from build123d import *

# Parameters (mm, degrees)
SCHIZZO1_R                   = 225
ESTRUSIONE_ESTRUSIONE1_DEPTH = 18
TAGLIO_ESTRUSIONE3_DEPTH     = 56
TAGLIO_ESTRUSIONE4_DEPTH     = 110


with BuildPart() as part:
    # Schizzo1 → Estrusione-Estrusione1 (new body)
    with BuildSketch(Plane.XY):
        Circle(SCHIZZO1_R)
    extrude(amount=ESTRUSIONE_ESTRUSIONE1_DEPTH)

    # Schizzo1<7> → Taglio-Estrusione3 (cut)
    with BuildSketch(Plane.XY):
        with BuildLine():
            Line((-11.65, 168.428927822), (-6.35, 168.428927822))
            ThreePointArc((-6.35, 168.428927822), (-3.175, 171.603927822), (0, 168.428927822))
            Line((0, 168.428927822), (0, 157.428927822))
            Line((0, 157.428927822), (11, 157.428927822))
            ThreePointArc((11, 157.428927822), (14.175, 154.253927822), (11, 151.078927822))
            Line((11, 151.078927822), (11, 145.778927822))
            ThreePointArc((11, 145.778927822), (14.175, 142.603927822), (11, 139.428927822))
            Line((11, 139.428927822), (0, 139.428927822))
            Line((0, 139.428927822), (0, 128.428927822))
            ThreePointArc((0, 128.428927822), (-3.175, 125.253927822), (-6.35, 128.428927822))
            Line((-6.35, 128.428927822), (-11.65, 128.428927822))
            ThreePointArc((-11.65, 128.428927822), (-14.825, 125.253927822), (-18, 128.428927822))
            Line((-18, 128.428927822), (-18, 139.428927822))
            Line((-18, 139.428927822), (-29, 139.428927822))
            ThreePointArc((-29, 139.428927822), (-32.175, 142.603927822), (-29, 145.778927822))
            Line((-29, 145.778927822), (-29, 151.078927822))
            ThreePointArc((-29, 151.078927822), (-32.175, 154.253927822), (-29, 157.428927822))
            Line((-29, 157.428927822), (-18, 157.428927822))
            Line((-18, 157.428927822), (-18, 168.428927822))
            ThreePointArc((-18, 168.428927822), (-14.825, 171.603927822), (-11.65, 168.428927822))
        make_face()
    extrude(amount=TAGLIO_ESTRUSIONE3_DEPTH, mode=Mode.SUBTRACT)

    # Schizzo1<8> → Taglio-Estrusione4 (cut)
    with BuildSketch(Plane.XY):
        with BuildLine():
            Line((-70.097292154, -124.331072178), (-64.797292154, -124.331072178))
            ThreePointArc((-64.797292154, -124.331072178), (-61.622292154, -121.156072178), (-58.447292154, -124.331072178))
            Line((-58.447292154, -124.331072178), (-58.447292154, -142.331072178))
            ThreePointArc((-58.447292154, -142.331072178), (-61.622292154, -145.506072178), (-64.797292154, -142.331072178))
            Line((-64.797292154, -142.331072178), (-70.097292154, -142.331072178))
            ThreePointArc((-70.097292154, -142.331072178), (-73.272292154, -145.506072178), (-76.447292154, -142.331072178))
            Line((-76.447292154, -142.331072178), (-76.447292154, -124.331072178))
            ThreePointArc((-76.447292154, -124.331072178), (-73.272292154, -121.156072178), (-70.097292154, -124.331072178))
        make_face()
    extrude(amount=TAGLIO_ESTRUSIONE4_DEPTH, mode=Mode.SUBTRACT)


solid = part.part
Here's how the part is built. I have some questions about the finished solid (model axes, mm). A direction names the side the tool comes from. Round coordinates to 2 decimals unless told otherwise and drop trailing zeros. Write each loop counter-clockwise with the first axis right and the second up, starting at its lowest first coordinate (ties: lowest second). Pieces come first, ordered by that corner, then holes.
1. Suppose I cut it at A-A (z = 8.5). State how many separate pieces and enclosed holes the cut face has, and give its area (3 significant figures).
2. Will these pins go through, and if not, where does the flat tip stop? pin 1 Ø5.5 at (y, z) = (132.5, 12) entering from -X; pin 2 Ø6 at (x, z) = (-106.5, 7.5) entering from -Y; pin 3 Ø5.5 at (y, z) = (-129.5, 6.5) entering from -X.
3. I need wall thicknesses on L1, parallel to Y at x = -30.5, z = 11.25; L2, parallel to X at y = 6.5, z = 1.25; L3, parallel to X at y = -126, z = 9. Which ranges of each line are inside material? Lowest first, please.
4. For faces 1 (the flat face through (-3, 3, 18)), 2 (the flat face through (-23, 139.429, 9)), which set-ups out of +Z, -Z, +X, -X, +Y, -Y let a thin tool reach every point of the face, with its end or its side?
5. Suppose I cut it at B-B (y = 85). List the corners of the cut face in (x, z) for me.
6. If we mould it in two halves opening along X, with no side actions, what happens to faces 3 (the cylindrical face through (-224.782, 9.893, 8.874)), 4 (the flat face through (0, 134, 9)), 5 (the flat face through (-3, 3, 0))? For each: released by +X, released by -X, zero draft, split by the parting line, or undercut.
7. Suppose I cut it at C-C (x = 159.5). List the corners of the cut face in (y, z) for me.
Answer sheet:
1. separate pieces: 1
1. enclosed holes: 2
1. area: 157,000 mm2
2. pin 1: stops at x = -183.82
2. pin 2: stops at y = -199.78
2. pin 3: stops at x = -185.9
3. L1: y = -222.92 to 139.81, 145.4 to 151.46, 157.05 to 222.92
3. L2: x = -224.91 to 224.91
3. L3: x = -186.41 to -76.45, -58.45 to 186.41
4. face 1: +Z, +X, -X, +Y, -Y
4. face 2: +Z, -Z
5. outline: (-208.33, 0) - (208.33, 0) - (208.33, 18) - (-208.33, 18) - close
6. face 3: split by the parting line
6. face 4: undercut
6. face 5: zero draft
7. outline: (-158.7, 0) - (158.7, 0) - (158.7, 18) - (-158.7, 18) - close
